Read the model definition and answer for the solid it produces. Units are mm, in the model's axes. A direction names the side the tool comes from. Coordinates: 2 decimals unless noted, no trailing zeros. Loops run counter-clockwise (first coordinate to the right, second up) from the corner with the lowest first, then second, coordinate; pieces in that order, holes last.
Q1. Which of the six approach directions +Z, -Z, +X, -X, +Y, -Y give full straight-line access (tool end or side, diameter ignored) to faces 1 (the face through (25, 0, 55)), 2 (the face through (-1, -25, 32)), 3 (the face through (4, 0, 80)), 4 (the face through (-20, 0, 70))?
Q2. The mould has two halves that part along X. Classify faces 5 (the face through (-12, 0, 79)), 6 (the face through (0, 0, 75)), 7 (the face through (27, 0, 40)): pulls with the +X half, pulls with the -X half, needs draft (parallel to the pull), parting line crosses it, or undercut.
Q3. Flat-ended cylindrical pins translate along their axes: P1, Ø2.5, axis at x = -28.5, y = -2, coming from the +Z side; P2, Ø7.5, axis at y = 12, z = 81.5, coming from the -X side; P3, Ø10.5, axis at y = 11, z = 81, coming from the +X side. Find the tip coordinate at first contact, or state that the pin passes through.
Q4. Section A-A (y = -12) is taken. Give the vertices of the cut face in (x, z), then the cut area to 3 significant figures.
Q5. Section B-B (z = 23.5) is taken. Give the vertices of the cut face in (x, y).
Q6. Straight lines are drawn through the part: line 1 (X direction, y = 10, z = 57); line 2 (Z direction, x = 25.5, y = 12); line 3 (Z direction, x = -3.5, y = -3). For each, find the intervals that lie inside material, in ascending order.
Q7. Section C-C (x = -35) is taken. Give the vertices of the cut face in (y, z).
from build123d import *

# Parameters (mm, degrees)
F0_W      = 92
F0_H      = 50
F1_DEPTH  = 40
F2_SIZE2  = 32
F2_SIZE   = 16
F3_SIZE2  = 32
F3_SIZE   = 16
F5_W      = 50
F5_H      = 50
F6_DEPTH  = 30
F8_DEPTH  = 50
F9_W      = 8
F9_H      = 20
F10_DEPTH = 50.001


with BuildPart() as f1:
    # F0 (on Top) → F1 (new body)
    with BuildSketch(Plane.XY):
        Rectangle(F0_W, F0_H)
    extrude(amount=F1_DEPTH)

    # F2
    f2_edges = [f1.edges().sort_by_distance(p)[0] for p in [
        (46, 0, 40),
    ]]
    f2_side = f1.faces().sort_by_distance((0, 0, 40))[0]
    chamfer(f2_edges, length=F2_SIZE, length2=F2_SIZE2, reference=f2_side)

    # F3
    f3_edges = [f1.edges().sort_by_distance(p)[0] for p in [
        (-46, 0, 40),
    ]]
    f3_side = f1.faces().sort_by_distance((-8, 0, 40))[0]
    chamfer(f3_edges, length=F3_SIZE, length2=F3_SIZE2, reference=f3_side)

    # F5 (on face) → F6 (join)
    with BuildSketch(Plane.XY.offset(40)):
        Rectangle(F5_W, F5_H)
    extrude(amount=F6_DEPTH)

    # F7 (on face) → F8 (join)
    with BuildSketch(Plane.XZ.offset(25)):
        with BuildLine():
            Line((-15, 70), (15, 70))
            ThreePointArc((15, 70), (0, 85), (-15, 70))
        make_face()
    extrude(amount=-F8_DEPTH)

    # F9 (on face) → F10 (cut, through all)
    with BuildSketch(Plane.XZ.offset(25)):
        with Locations((0, 85)):
            Rectangle(F9_W, F9_H)
    extrude(amount=-F10_DEPTH, mode=Mode.SUBTRACT)


solid = f1.part
Numbers:
1. face 1: +Z, +X, +Y, -Y
1. face 2: +Z, -Z, +X, -X, -Y
1. face 3: +Z, +Y, -Y
1. face 4: +Z, -X, +Y, -Y
2. face 5: pulls with the -X half
2. face 6: undercut
2. face 7: needs draft
3. P1: stops at z = 40
3. P2: stops at x = -12.84
3. P3: stops at x = 13.85
4. outline: (-46, 0) - (46, 0) - (46, 8) - (30, 40) - (25, 40) - (25, 70) - (15, 70) arc R15 ccw to (4, 84.46) - (4, 75) - (-4, 75) - (-4, 84.46) arc R15 ccw to (-15, 70) - (-25, 70) - (-25, 40) - (-30, 40) - (-46, 8) - close
4. area: 4,940 mm2
5. outline: (-38.25, -25) - (38.25, -25) - (38.25, 25) - (-38.25, 25) - close
6. line 1: x = -25 to 25
6. line 2: z = 0 to 40
6. line 3: z = 0 to 75
7. outline: (-25, 0) - (25, 0) - (25, 30) - (-25, 30) - close
